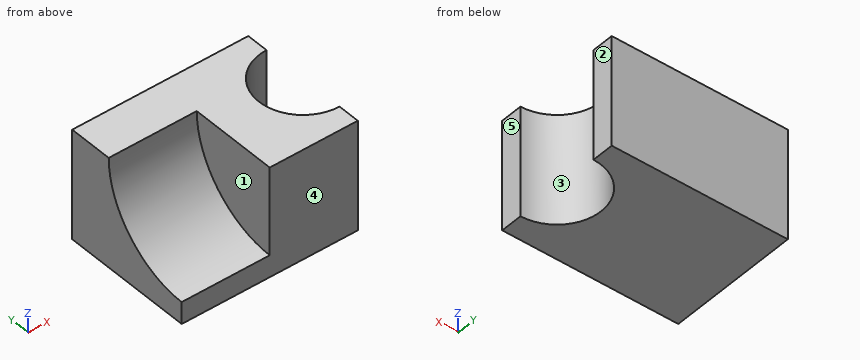
```python
from build123d import *

# Parameters (mm, degrees)
F0_W     = 101.6
F0_H     = 63.5
F1_DEPTH = 76.2
F3_DEPTH = 63.5
F5_DEPTH = 50.8


with BuildPart() as f1:
    # F0 (on Front) → F1 (new body)
    with BuildSketch(Plane.XZ):
        with Locations((-3.26282, -0.310746)):
            Rectangle(F0_W, F0_H)
    extrude(amount=F1_DEPTH)

    # F2 (on face) → F3 (cut)
    with BuildSketch(Plane.XY.offset(31.439254)):
        with BuildLine():
            Line((47.53718, -63.5), (47.53718, -12.7))
            ThreePointArc((47.53718, -12.7), (22.13718, -38.1), (47.53718, -63.5))
        make_face()
    extrude(amount=-F3_DEPTH, mode=Mode.SUBTRACT)

    # F4 (on face) → F5 (cut)
    with BuildSketch(Plane(origin=(-54.06282, 0, 0), x_dir=(0, -1, 0), z_dir=(-1, 0, 0))):
        with BuildLine():
            Line((76.2, 31.439254), (25.4, 31.439254))
            ThreePointArc((25.4, 31.439254), (40.278976, -4.481771), (76.2, -19.360746))
            Line((76.2, -19.360746), (76.2, 31.439254))
        make_face()
    extrude(amount=-F5_DEPTH, mode=Mode.SUBTRACT)


solid = f1.part
```
Geometry check sheet. Reference: the model listing, model coordinates, mm. Face numbers are marked on the shaded views. A direction names the side the tool comes from. Coordinates: 2 decimals unless noted, no trailing zeros. Order: outer loops, then holes, each group sorted by start corner. A loop starts at its lowest first (then second) coordinate and runs counter-clockwise, first axis right, second up.
Q1. Sectioned sample at B-B on x = -24. Record the cut outline in (y, z).
Reply:
outline: (-76.2, -32.06) - (0, -32.06) - (0, 31.44) - (-25.4, 31.44) arc R50.8 cw to (-76.2, -19.36) - close
Q2. Sectioned sample at D-D on y = -38.1. Record the cut outline in (x, z), and give its area (3 significant figures).
Reply:
outline: (-54.06, -32.06) - (22.14, -32.06) - (22.14, 31.44) - (-3.26, 31.44) - (-3.26, -2.16) - (-54.06, -2.16) - close
area: 3,130 mm2
Q3. Sectioned sample at A-A on x = 40.5. Record the cut outline in (y, z), and give its area (3 significant figures).
Reply:
outline: (-76.2, -32.06) - (-62.51, -32.06) - (-62.51, 31.44) - (-76.2, 31.44) - close; (-13.69, -32.06) - (0, -32.06) - (0, 31.44) - (-13.69, 31.44) - close
area: 1,740 mm2
Q4. Sectioned sample at C-C on z = -8. Record the cut outline in (x, y), and give its area (3 significant figures).
Reply:
outline: (-54.06, -44.18) - (-3.26, -44.18) - (-3.26, -76.2) - (47.54, -76.2) - (47.54, -63.5) arc R25.4 cw to (47.54, -12.7) - (47.54, 0) - (-54.06, 0) - close
area: 5,100 mm2
Q5. Depth check by flat-ended pin: pin 1 Ø1.5 at (x, z) = (10.5, -20.5) entering from +Y; pin 2 Ø2 at (x, y) = (-8, -66) entering from +Z; pin 3 Ø10 at (y, z) = (-52.5, -1) entering from -X; pin 4 Ø5 at (x, z) = (-7, -5.5) entering from -Y. Enter the tip coordinate at first touch or a pass-through.
Reply:
pin 1: stops at y = 0
pin 2: stops at z = -18.11
pin 3: stops at x = -3.26
pin 4: stops at y = -44.18
Q6. Thickness scan on probe 1 along Y at (x, z) = (34.5, -11.5); probe 2 along X at (y, z) = (-68, -13); probe 3 along X at (y, z) = (-38, 15.5). Record the ranges inside material, lowest first.
Reply:
probe 1: y = -76.2 to -59.9, -16.3 to 0
probe 2: x = -3.26 to 47.54
probe 3: x = -3.26 to 22.14
Q7. Draft check along Y on the marked faces 3, 4 and 5. Enter one of: released by +Y, released by -Y, zero draft, split by the parting line, or undercut.
Reply:
face 3: undercut
face 4: released by -Y
face 5: zero draft
Q8. Tool access check on the marked faces 1 and 2. Record the directions out of +Z, -Z, +X, -X, +Y, -Y that give a thin tool (end or side, any length) a straight path to the whole face; none if there is none.
Reply:
face 1: +Z, -X, -Y
face 2: +Z, -Z, +X, +Y, -Y
